Part model, mm, in its own coordinate system. A direction names the side the tool comes from. Coordinates: 2 decimals unless noted, no trailing zeros. Loops run counter-clockwise (first coordinate to the right, second up) from the corner with the lowest first, then second, coordinate; pieces in that order, holes last. Notation, with made-up numbers: (73, 53.5) - (82, 53.5) arc R35 cw to (82, 85.5) - close; hole circle Ø9 at (72.25, 13). An arc over 180 degrees is marked (long way). Use a Markdown table: item, result. Add a question column.
1) Drop flat-ended pins along their axis: P1, Ø3, axis at x = -86.5, z = 5.5, coming from the +Y side; P2, Ø8, axis at x = -123.5, y = -86.5, coming from the -Z side; P3, Ø10, axis at x = -64.5, y = -10.5, coming from the -Z side; P4, Ø9, axis at x = 125.14, y = -87.52, coming from the -Z side. Give the stop position or say it passes through.
2) Band-saw the part on D-D (x = 103). Give the cut face in (y, z).
3) Tool access for faces 1 (the face through (-125, -93, 5)), 2 (the face through (-2.38, -10.74, 5.07)), 3 (the face through (-1, -15, 5)), 4 (the face through (-2.5, 2.8, -5)), 5 (the face through (-11, -13, 10)): list every direction of +Z, -Z, +X, -X, +Y, -Y with a clear straight run to the whole face (end or side of a thin tool).
4) Band-saw the part on C-C (x = -33). Give the cut face in (y, z), plus the area to 3 significant figures.
5) Pull direction Y, two halves, no side cores. Call faces 6 (the face through (-132.93, -100.34, 4.93)), 7 (the face through (-114.713, -39.449, 4.93)), 8 (the face through (-123.45, -74.63, 2.46)): +Y half, -Y half, draft (parallel to the pull), parting line (faces both ways), or undercut.
6) Band-saw the part on A-A (x = 0). Give the cut face in (y, z), plus the area to 3 significant figures.
7) Probe probe 1 along Y at (x, z) = (-0.5, 9); probe 2 along Y at (x, z) = (0, -1.8); probe 3 along X at (y, z) = (2.5, -1.5). List the from-to ranges inside material, lowest first. Write a range as [from, to].
8) Band-saw the part on B-B (y = -18.5). Give the cut face in (x, z), plus the area to 3 significant figures.
from build123d import *

# Parameters (mm, degrees)
SKETCH1_R           = 1.75
BOSS_EXTRUDE1_DEPTH = 10
SKETCH2_R           = 11
SKETCH2_R_2         = 5
CUT_EXTRUDE1_DEPTH  = 10
SKETCH3_R           = 12
BOSS_EXTRUDE2_DEPTH = 5
SKETCH4_R           = 13
CUT_EXTRUDE2_DEPTH  = 5
SKETCH5_R           = 3.5
CUT_EXTRUDE3_DEPTH  = 175.285919969


with BuildPart() as part:
    # Sketch1 → Boss-Extrude1 (new body)
    with BuildSketch(Plane.XY):
        with BuildLine():
            Line((65.95591629, 15), (-65.95591629, 15))
            ThreePointArc((-65.95591629, 15), (-80.95591629, 10.980762114), (-91.936678404, 0))
            Line((-91.936678404, 0), (-138.135251983, -80.018276676))
            ThreePointArc((-138.135251983, -80.018276676), (-132.644870926, -100.508657733), (-112.154489869, -95.018276676))
            Line((-112.154489869, -95.018276676), (-65.95591629, -15))
            Line((-65.95591629, -15), (65.95591629, -15))
            Line((65.95591629, -15), (112.154489869, -95.018276676))
            ThreePointArc((112.154489869, -95.018276676), (132.644870926, -100.508657733), (138.135251983, -80.018276676))
            Line((138.135251983, -80.018276676), (91.936678404, 0))
            ThreePointArc((91.936678404, 0), (80.95591629, 10.980762114), (65.95591629, 15))
        make_face()
        with Locations((-133.644870926, -87.518276676)):
            Circle(SKETCH1_R, mode=Mode.SUBTRACT)
        with Locations((-116.644870926, -87.518276676)):
            Circle(SKETCH1_R, mode=Mode.SUBTRACT)
    extrude(amount=BOSS_EXTRUDE1_DEPTH)

    # Sketch2 → Cut-Extrude1 (cut)
    with BuildSketch(Plane.XY.offset(10)):
        Circle(SKETCH2_R)
        with Locations((-125.144870926, -87.518276676)):
            Circle(SKETCH2_R_2)
        with Locations((125.144870926, -87.518276676)):
            Circle(SKETCH2_R_2)
    extrude(amount=-CUT_EXTRUDE1_DEPTH, mode=Mode.SUBTRACT)

    # Sketch3 → Boss-Extrude2 (add)
    with BuildSketch(Plane(origin=(0, 0, 0), x_dir=(-1, 0, 0), z_dir=(0, 0, -1))):
        Circle(SKETCH3_R)
    extrude(amount=BOSS_EXTRUDE2_DEPTH)

    # Sketch4 → Cut-Extrude2 (cut)
    with BuildSketch(Plane(origin=(0, 0, 0), x_dir=(-1, 0, 0), z_dir=(0, 0, -1))):
        with Locations((125.144870926, -87.518276676)):
            Circle(SKETCH4_R)
    extrude(amount=-CUT_EXTRUDE2_DEPTH, mode=Mode.SUBTRACT)

    # Sketch5 → Cut-Extrude3 (cut, through all)
    with BuildSketch(Plane.XY.offset(10)):
        Circle(SKETCH5_R)
    extrude(amount=-CUT_EXTRUDE3_DEPTH, mode=Mode.SUBTRACT)


solid = part.part
Answer block:
| question | item | result |
|---|---|---|
| 1 | P1 | y = 8.18 |
| 1 | P2 | z = 5 |
| 1 | P3 | z = 0 |
| 1 | P4 | through |
| 2 | outline | (-79.16, 0) - (-19.16, 0) - (-19.16, 10) - (-79.16, 10) - close |
| 3 | face 1 | -Z |
| 3 | face 2 | +Z |
| 3 | face 3 | +Z, -Z, -Y |
| 3 | face 4 | -Z, +X, -X, +Y, -Y |
| 3 | face 5 | +Z, +X, -X, +Y, -Y |
| 4 | outline | (-15, 0) - (15, 0) - (15, 10) - (-15, 10) - close |
| 4 | area | 300 mm2 |
| 5 | face 6 | parting line |
| 5 | face 7 | +Y half |
| 5 | face 8 | undercut |
| 6 | outline | (-15, 0) - (-12, 0) - (-12, -5) - (-3.5, -5) - (-3.5, 0) - (-11, 0) - (-11, 10) - (-15, 10) - close; (3.5, -5) - (12, -5) - (12, 0) - (15, 0) - (15, 10) - (11, 10) - (11, 0) - (3.5, 0) - close |
| 6 | area | 165 mm2 |
| 7 | probe 1 | [-15, -10.99], [10.99, 15] |
| 7 | probe 2 | [-12, -3.5], [3.5, 12] |
| 7 | probe 3 | [-11.74, -2.45], [2.45, 11.74] |
| 8 | outline | (-102.62, 0) - (-67.98, 0) - (-67.98, 10) - (-102.62, 10) - close; (67.98, 0) - (102.62, 0) - (102.62, 10) - (67.98, 10) - close |
| 8 | area | 693 mm2 |
